Verification items for the finished model (mm, model axes). A direction names the side the tool comes from. Give positions to 0.01 mm unless a question says otherwise; leave off trailing zeros. Order: outer loops, then holes, each group sorted by start corner. A loop starts at its lowest first (then second) coordinate and runs counter-clockwise, first axis right, second up. Notation, with made-up numbers: (3.25, 45.25) -> (62.25, 45.25) arc R25 cw to (62.25, 60.25) -> close; hole circle Ø11 at (15, -9). An arc over 180 degrees is marked (long way). One line per question, with ' | ' between items. Start each with the question number.
Q1. Section check D-D on z = 3.25. Record the cut outline in (x, y), plus the area to 3 significant figures.
Q2. Material ranges on probe 1 along Y at (x, z) = (18.5, 16); probe 2 along Z at (x, y) = (15.5, 18.5); probe 3 along Z at (x, y) = (24, 24.5), recorded low to high. Write a range as [from, to].
Q3. Access from +Z, -Z, +X, -X, +Y, -Y to the whole of each face (thin tool, end or side, straight path). Record for faces 1 (the cylindrical face through (31.01, 0.6, 19.43)), 2 (the cylindrical face through (24.21, 7.25, 17.78)), 3 (the flat face through (30, 15, 13)).
Q4. Mould release check, pull along X, two halves, no side actions. Record for faces 4 (the flat face through (20, 20, 5)), 5 (the flat face through (23.6, 24.85, 20)), 6 (the flat face through (24, 25, 13)), 7 (the cylindrical face through (21.07, 33.4, 8.87)): released by +X, released by -X, zero draft, split by the parting line, or undercut.
Q5. Section check B-B on y = 5.5. Record the cut outline in (x, z).
Q6. Section check C-C on x = 10.5. Record the cut outline in (y, z), plus the area to 3 significant figures.
Q7. Section check A-A on z = 9.75. Record the cut outline in (x, y), plus the area to 3 significant figures.
Q8. Go/stop test with flat-tipped pins: pin 1 (5 mm diameter, centred on x = 13, y = 24, fed in from +Z); pin 2 (1.3 mm diameter, centred on x = 20.5, z = 17.5, fed in from +Y); pin 3 (1 mm diameter, centred on x = 15.5, z = 12.5, fed in from -Y); pin 4 (7.5 mm diameter, centred on y = 9, z = 9.5, fed in from -X). Record where each tip stops, or that it passes through.
from build123d import *

# Parameters (mm, degrees)
F0_W      = 34
F0_H      = 34
F1_DEPTH  = 20
F3_DEPTH  = 15
F4_SIZE   = 1
F6_W      = 20.5
F6_H      = 5.5
F7_DEPTH  = 20.001
F8_R      = 2
F9_R      = 2
F10_DEPTH = 4.5
F11_R     = 3.1
F12_DEPTH = 15.501
F13_R     = 1
F14_SIZE  = 15
F15_R     = 5


with BuildPart() as f1:
    # F0 (on Top) → F1 (new body)
    with BuildSketch(Plane.XY):
        with Locations((17, 17)):
            Rectangle(F0_W, F0_H)
    extrude(amount=F1_DEPTH)

    # F2 (on face) → F3 (cut)
    with BuildSketch(Plane.XY.offset(20)):
        Polygon((24.5, 0), (30, 0), (30, 30), (24.5, 30), (24.5, 24.5), (0, 24.5), (0, 19), (24.5, 19), align=None)
    extrude(amount=-F3_DEPTH, mode=Mode.SUBTRACT)

    # F4
    f4_edges = [f1.edges().sort_by_distance(p)[0] for p in [
        (24.5, 24.5, 12.5),
        (24.5, 19, 12.5),
    ]]
    chamfer(f4_edges, length=F4_SIZE)

    # F6 (on face) → F7 (cut, through all)
    with BuildSketch(Plane.XY.offset(20)):
        with Locations((10.25, 31.25)):
            Rectangle(F6_W, F6_H)
    extrude(amount=-F7_DEPTH, mode=Mode.SUBTRACT)

    # F8
    f8_edges = [f1.edges().sort_by_distance(p)[0] for p in [
        (0, 28.5, 10),
        (20.5, 28.5, 10),
        (20.5, 34, 10),
        (34, 34, 10),
        (34, 0, 10),
    ]]
    fillet(f8_edges, radius=F8_R)

    # F9
    f9_edges = [f1.edges().sort_by_distance(p)[0] for p in [
        (31, 0, 20),
    ]]
    fillet(f9_edges, radius=F9_R)

    # F5 (on face) → F10 (cut)
    with BuildSketch(Plane.XY.offset(20)):
        with BuildLine():
            Line((13.0466991411, 20.6966991411), (13.0466991411, 13.1966991411))
            ThreePointArc((13.0466991411, 13.1966991411), (14.7015458274, 9.2015458274), (18.6966991411, 7.5466991411))
            Line((18.6966991411, 7.5466991411), (26.0466991411, 7.5466991411))
            Line((26.0466991411, 7.5466991411), (26.0466991411, 20.6966991411))
            Line((26.0466991411, 20.6966991411), (13.0466991411, 20.6966991411))
        make_face()
    extrude(amount=-F10_DEPTH, mode=Mode.SUBTRACT)

    # F11 (on face) → F12 (cut, through all)
    with BuildSketch(Plane.XY.offset(15.5)):
        with Locations((18.6966991411, 13.1966991411)):
            Circle(F11_R)
    extrude(amount=-F12_DEPTH, mode=Mode.SUBTRACT)

    # F13
    f13_edges = [f1.edges().sort_by_distance(p)[0] for p in [
        (13.046699, 19, 17.75),
        (24.5, 7.546699, 17.75),
    ]]
    fillet(f13_edges, radius=F13_R)

    # F14
    f14_edges = [f1.edges().sort_by_distance(p)[0] for p in [
        (0, 0, 10),
    ]]
    chamfer(f14_edges, length=F14_SIZE)

    # F15
    f15_edges = [f1.edges().sort_by_distance(p)[0] for p in [
        (0, 15, 10),
        (15, 0, 10),
    ]]
    fillet(f15_edges, radius=F15_R)


solid = f1.part
Filled in:
1) outline: (0, 17.07) arc R5 ccw to (1.46, 13.54) -> (13.54, 1.46) arc R5 ccw to (17.07, 0) -> (32, 0) arc R2 ccw to (34, 2) -> (34, 32) arc R2 ccw to (32, 34) -> (22.5, 34) arc R2 ccw to (20.5, 32) -> (20.5, 30.5) arc R2 cw to (18.5, 28.5) -> (2, 28.5) arc R2 ccw to (0, 26.5) -> close; hole circle Ø6.2 at (18.7, 13.2) | area: 897 mm²
2) probe 1: [0, 7.55], [24.5, 28.5] | probe 2: [0, 15.5] | probe 3: [0, 5]
3) face 1: +Z, +X, -Y | face 2: +Z | face 3: +Z, -Y
4) face 4: undercut | face 5: zero draft | face 6: undercut | face 7: released by -X
5) outline: (9.5, 0) -> (34, 0) -> (34, 18) arc R2 ccw to (32, 20) -> (30, 20) -> (30, 5) -> (24.5, 5) -> (24.5, 20) -> (9.5, 20) -> close
6) outline: (4.5, 0) -> (28.5, 0) -> (28.5, 18) arc R2 ccw to (26.5, 20) -> (24.5, 20) -> (24.5, 5) -> (19, 5) -> (19, 20) -> (4.5, 20) -> close | area: 397 mm²
7) outline: (0, 17.07) arc R5 ccw to (1.46, 13.54) -> (13.54, 1.46) arc R5 ccw to (17.07, 0) -> (24.5, 0) -> (24.5, 18) -> (23.5, 19) -> (0, 19) -> close; (0, 24.5) -> (23.5, 24.5) -> (24.5, 25.5) -> (24.5, 30) -> (30, 30) -> (30, 0) -> (32, 0) arc R2 ccw to (34, 2) -> (34, 32) arc R2 ccw to (32, 34) -> (22.5, 34) arc R2 ccw to (20.5, 32) -> (20.5, 30.5) arc R2 cw to (18.5, 28.5) -> (2, 28.5) arc R2 ccw to (0, 26.5) -> close; hole circle Ø6.2 at (18.7, 13.2) | area: 596 mm²
8) pin 1: z = 20 | pin 2: y = 33.48 | pin 3: y = 0.12 | pin 4: x = 2.25
